Part model, mm, in its own coordinate system. A direction names the side the tool comes from. Coordinates: 2 decimals unless noted, no trailing zeros. Loops run counter-clockwise (first coordinate to the right, second up) from the corner with the lowest first, then second, coordinate; pieces in that order, holes last. Notation, with made-up numbers: (69, 14) - (78, 14) arc R27 cw to (78, 33) - close; hole circle Ø5 at (4.5, 19). An arc over 180 degrees is marked (long way). Answer as CSV lines item,"result".
from build123d import *

# Parameters (mm, degrees)
SKETCH_3_W             = 58
SKETCH_3_H             = 37
EXTRUDE_1_DEPTH        = 2
SKETCH_4_W             = 58
SKETCH_4_H             = 2
EXTRUDE_2_DEPTH        = 23.5
SKETCH_5_W             = 8
SKETCH_5_H             = 2
EXTRUDE_3_DEPTH        = 23.5
PATTERN_LINEAR_1_COUNT = 2
PATTERN_LINEAR_1_PITCH = 50
SKETCH_6_W             = 6
SKETCH_6_H             = 6
CUT_EXTRUDE_1_DEPTH    = 44.950905628
PATTERN_LINEAR_2_COUNT = 2
PATTERN_LINEAR_2_PITCH = 52
CUT_EXTRUDE_2_DEPTH    = 23.5
CUT_EXTRUDE_3_DEPTH    = 23.5
SKETCH_9_R             = 2
SKETCH_9_R_2           = 4
SKETCH_9_R_3           = 1.5
CUT_EXTRUDE_4_DEPTH    = 23.5
SKETCH_11_R            = 2.447120917
SKETCH_11_R_2          = 1.5
CUT_EXTRUDE_5_DEPTH    = 53.925233976
FILLET_1_R             = 2
SKETCH_12_R            = 2
CUT_EXTRUDE_6_DEPTH    = 23.5


with BuildPart() as part:
    # 草图3 → 凸台-拉伸1 (new body)
    with BuildSketch(Plane.XY):
        with Locations((-1.42746114, 2.797927461)):
            Rectangle(SKETCH_3_W, SKETCH_3_H)
    extrude(amount=EXTRUDE_1_DEPTH)

    # 草图4 → 凸台-拉伸2 (add)
    with BuildSketch(Plane.XY.offset(2)):
        with Locations((-1.42746114, -14.702072539)):
            Rectangle(SKETCH_4_W, SKETCH_4_H)
    extrude(amount=EXTRUDE_2_DEPTH)

    # 草图5 → 凸台-拉伸3 (add)
    with BuildSketch(Plane.XY.offset(2)):
        with Locations((-26.42746114, 15.297927461)):
            Rectangle(SKETCH_5_W, SKETCH_5_H)
    extrude_3 = extrude(amount=EXTRUDE_3_DEPTH)

    # 阵列(线性)1: 凸台-拉伸3 ×2
    with Locations(*[(i * PATTERN_LINEAR_1_PITCH, 0, 0) for i in range(1, PATTERN_LINEAR_1_COUNT)]):
        add(extrude_3)

    # 草图6 → 切除-拉伸1 (cut, symmetric)
    with BuildSketch(Plane.XY.offset(2)):
        with Locations((-27.42746114, -12.702072539)):
            Rectangle(SKETCH_6_W, SKETCH_6_H)
    cut_extrude_1 = extrude(amount=CUT_EXTRUDE_1_DEPTH, both=True, mode=Mode.SUBTRACT)

    # 阵列(线性)2: 切除-拉伸1 ×2
    with Locations(*[(i * PATTERN_LINEAR_2_PITCH, 0, 0) for i in range(1, PATTERN_LINEAR_2_COUNT)]):
        add(cut_extrude_1, mode=Mode.SUBTRACT)

    # 草图7 → 切除-拉伸2 (cut)
    with BuildSketch(Plane.XY.offset(2)):
        Polygon((-30.42746114, 21.297927461), (-30.42746114, 16.297927461), (-22.42746114, 16.297927461), (-22.42746114, 14.297927461), (-22.42746114, 12.297927461), (-20.42746114, 12.297927461), (-20.42746114, 21.297927461), align=None)
    extrude(amount=-CUT_EXTRUDE_2_DEPTH, mode=Mode.SUBTRACT)

    # 草图8 → 切除-拉伸3 (cut)
    with BuildSketch(Plane.XY.offset(2)):
        Polygon((27.57253886, 16.297927461), (27.57253886, 21.297927461), (17.57253886, 21.297927461), (17.57253886, 12.297927461), (19.57253886, 12.297927461), (19.57253886, 16.297927461), align=None)
    extrude(amount=-CUT_EXTRUDE_3_DEPTH, mode=Mode.SUBTRACT)

    # 草图9 → 切除-拉伸4 (cut)
    with BuildSketch(Plane.XY.offset(2)):
        with Locations((-27.42746114, 6.297927461)):
            Circle(SKETCH_9_R)
        with Locations((-27.42746114, -3.702072539)):
            Circle(SKETCH_9_R)
        with Locations((-11.92746114, 6.297927461)):
            Circle(SKETCH_9_R_2)
        with Locations((-1.42746114, -3.702072539)):
            Circle(SKETCH_9_R_2)
        with Locations((-1.42746114, 3.297927461)):
            Circle(SKETCH_9_R_3)
        with Locations((-1.42746114, -10.702072539)):
            Circle(SKETCH_9_R_3)
        with Locations((-11.92746114, -0.702072539)):
            Circle(SKETCH_9_R_3)
        with Locations((-11.92746114, 13.297927461)):
            Circle(SKETCH_9_R_3)
        with Locations((-18.92746114, 6.297927461)):
            Circle(SKETCH_9_R_3)
        with Locations((-4.92746114, 6.297927461)):
            Circle(SKETCH_9_R_3)
        with Locations((-8.42746114, -3.702072539)):
            Circle(SKETCH_9_R_3)
        with Locations((5.57253886, -3.702072539)):
            Circle(SKETCH_9_R_3)
        with Locations((9.07253886, 13.297927461)):
            Circle(SKETCH_9_R_3)
        with Locations((2.07253886, 6.297927461)):
            Circle(SKETCH_9_R_3)
        with Locations((9.07253886, -0.702072539)):
            Circle(SKETCH_9_R_3)
        with Locations((9.07253886, 6.297927461)):
            Circle(SKETCH_9_R_2)
        with Locations((16.07253886, 6.297927461)):
            Circle(SKETCH_9_R_3)
        with Locations((24.57253886, -3.702072539)):
            Circle(SKETCH_9_R)
        with Locations((24.57253886, 6.297927461)):
            Circle(SKETCH_9_R)
    extrude(amount=-CUT_EXTRUDE_4_DEPTH, mode=Mode.SUBTRACT)

    # 草图11 → 切除-拉伸5 (cut, through all)
    with BuildSketch(Plane(origin=(0, -13.702072539, 0), x_dir=(1, 0, 0), z_dir=(0, 1, 0))):
        with Locations(Location((-11.92746114, -13.75, 0), (0, 0, 270))):
            Circle(SKETCH_11_R)
        with Locations(Location((-18.92746114, -13.75, 0), (0, 0, 270))):
            Circle(SKETCH_11_R_2)
        with Locations(Location((-11.92746114, -20.75, 0), (0, 0, 270))):
            Circle(SKETCH_11_R_2)
        with Locations(Location((-4.92746114, -13.75, 0), (0, 0, 270))):
            Circle(SKETCH_11_R_2)
        with Locations(Location((-11.92746114, -6.75, 0), (0, 0, 270))):
            Circle(SKETCH_11_R_2)
        with Locations(Location((9.07253886, -20.75, 0), (0, 0, 90))):
            Circle(SKETCH_11_R_2)
        with Locations(Location((2.07253886, -13.75, 0), (0, 0, 90))):
            Circle(SKETCH_11_R_2)
        with Locations(Location((9.07253886, -6.75, 0), (0, 0, 90))):
            Circle(SKETCH_11_R_2)
        with Locations(Location((9.07253886, -13.75, 0), (0, 0, 90))):
            Circle(SKETCH_11_R)
        with Locations(Location((16.07253886, -13.75, 0), (0, 0, 90))):
            Circle(SKETCH_11_R_2)
    extrude(amount=-CUT_EXTRUDE_5_DEPTH, mode=Mode.SUBTRACT)

    # 圆角1
    fillet_1_edges = [part.edges().sort_by_distance(p)[0] for p in [
        (-1.42746114, -15.702072539, 0),
        (-30.42746114, -9.702072539, 1),
        (27.57253886, -9.702072539, 1),
        (-20.42746114, 21.297927461, 1),
        (17.57253886, 21.297927461, 1),
        (23.57253886, 16.297927461, 0),
        (-26.42746114, 16.297927461, 0),
        (27.57253886, 15.297927461, 25.5),
        (19.57253886, 15.297927461, 25.5),
        (21.57253886, -14.702072539, 25.5),
        (-24.42746114, -14.702072539, 25.5),
        (-22.42746114, 15.297927461, 25.5),
        (-30.42746114, 15.297927461, 25.5),
    ]]
    fillet(fillet_1_edges, radius=FILLET_1_R)

    # 草图12 → 切除-拉伸6 (cut)
    with BuildSketch(Plane(origin=(0, 16.297927461, 0), x_dir=(1, 0, 0), z_dir=(0, 1, 0))):
        with Locations(Location((-26.42746114, -19.25, 0), (0, 0, 270))):
            Circle(SKETCH_12_R)
        with Locations(Location((-26.42746114, -8.25, 0), (0, 0, 270))):
            Circle(SKETCH_12_R)
        with Locations(Location((23.57253886, -19.25, 0), (0, 0, 270))):
            Circle(SKETCH_12_R)
        with Locations(Location((23.57253886, -8.25, 0), (0, 0, 270))):
            Circle(SKETCH_12_R)
    extrude(amount=-CUT_EXTRUDE_6_DEPTH, mode=Mode.SUBTRACT)


solid = part.part
Q1. Two-plate mould, pull along Y, no slides. Class faces 4 (the face through (-1.11, -15.1, 0.57)), 5 (the face through (10.537, -14.688, 7.075)), 6 (the face through (-17.497, 6.748, 1.014)): released by +Y, released by -Y, zero draft, split by the parting line, or undercut.
Results:
face 4,"released by -Y"
face 5,"zero draft"
face 6,"undercut"
Q2. Flat gauge pins, fed straight in: pin 1 (6.5 mm diameter, centred on y = -14, z = 10, fed in from +X); pin 2 (3 mm diameter, centred on x = 9.07, z = 13.75, fed in from +Y); pin 3 (1 mm diameter, centred on x = -1.5, y = 8.5, fed in from +Z); pin 4 (0.6 mm diameter, centred on x = -21.5, z = 1, fed in from +Y). Where does each tip first touch, or does it go through?
Results:
pin 1,"stops at x = 21.57"
pin 2,"passes through"
pin 3,"stops at z = 2"
pin 4,"stops at y = 12.3"
Q3. Saw through at C-C (z = 13.75). Count the separate pieces of the cut face and the enclosed holes in it, then the cut area to 3 significant figures.
Results:
separate pieces,"9"
enclosed holes,"0"
area,"80.4 mm^2"
Q4. Wall check: L1, parallel to X at y = -15.2, z = 6.75; L2, parallel to Z at x = -22, y = -0.5; L3, parallel to Y at x = -25.5, z = 22. Give the ranges that are in metal, low to high.
Results:
L1,"x = -24.43 to -13.43, -10.43 to 7.57, 10.57 to 21.57"
L2,"z = 0 to 2"
L3,"y = 14.3 to 16.3"
Q5. Saw through at B-B (x = -21.5). Give the cut face in (y, z), then the cut area to 3 significant figures.
Results:
outline,"(-15.7, 2) arc R2 ccw to (-13.7, 0) - (12.3, 0) - (12.3, 2) - (-13.7, 2) - (-13.7, 25.5) - (-15.7, 25.5) - close"
area,"102 mm^2"
Q6. Saw through at A-A (z = 7.25). Give the cut face in (x, y), then the cut area to 3 significant figures.
Results:
outline,"(-30.43, 14.3) - (-28.16, 14.3) - (-28.16, 16.3) - (-30.43, 16.3) - close; (-24.7, 14.3) - (-22.43, 14.3) - (-22.43, 16.3) - (-24.7, 16.3) - close; (-24.43, -15.7) - (-13.34, -15.7) - (-13.34, -13.7) - (-24.43, -13.7) - close; (-10.51, -15.7) - (7.66, -15.7) - (7.66, -13.7) - (-10.51, -13.7) - close; (10.49, -15.7) - (21.57, -15.7) - (21.57, -13.7) - (10.49, -13.7) - close; (19.57, 14.3) - (21.84, 14.3) - (21.84, 16.3) - (19.57, 16.3) - close; (25.3, 14.3) - (27.57, 14.3) - (27.57, 16.3) - (25.3, 16.3) - close"
area,"98.8 mm^2"
Q7. Which spindle directions (+Z, -Z, +X, -X, +Y, -Y) get a long thin tool onto all of the face, cutting with end or side? Do faces 1 (the face through (24, 14.298, 14)), 2 (the face through (-23, 15.3, 24.9)), 3 (the face through (21, -14.7, 24.9)). Say none if no direction does.
Results:
face 1,"+Z, +X, -X"
face 2,"+Z, +Y"
face 3,"+Z, +X, -Y"
